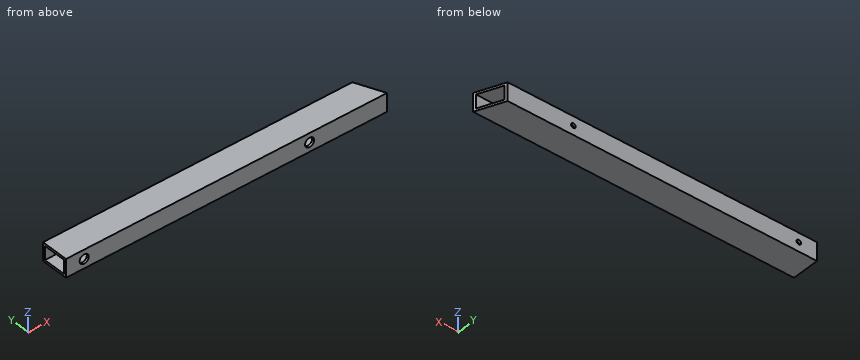
```python
from build123d import *

# Parameters (mm, degrees)
SKETCH1_W                 = 25.4
SKETCH1_H                 = 38.1
SKETCH1_W_2               = 19.05
SKETCH1_H_2               = 31.75
BEAM_DEPTH                = 447.675
MITER_CUT_DEPTH           = 449.799474292
SKETCH4_R                 = 3.175
BOLT_CLEARANCE_HOLE_DEPTH = 450.472808549
SKETCH5_R                 = 6.35
CLEARANCE_HOLE_DEPTH      = 12.7


with BuildPart() as part:
    # Sketch1 → beam (new body)
    with BuildSketch(Plane(origin=(0, 0, 0), x_dir=(0, 0, -1), z_dir=(1, 0, 0))):
        Rectangle(SKETCH1_W, SKETCH1_H)
        Rectangle(SKETCH1_W_2, SKETCH1_H_2, mode=Mode.SUBTRACT)
    extrude(amount=-BEAM_DEPTH)

    # Sketch2 → miter cut (cut, through all)
    with BuildSketch(Plane.XY.offset(12.7)):
        Polygon((0, -19.05), (-16.172490498, 19.05), (0, 19.05), align=None)
    extrude(amount=-MITER_CUT_DEPTH, mode=Mode.SUBTRACT)

    # Sketch4 → bolt clearance hole (cut, through all)
    with BuildSketch(Plane(origin=(0, 19.05, 0), x_dir=(1, 0, 0), z_dir=(0, 1, 0))):
        with Locations(Location((-422.275, 0, 0), (0, 0, 270))):
            Circle(SKETCH4_R)
        with Locations(Location((-107.95, 0, 0), (0, 0, 270))):
            Circle(SKETCH4_R)
    extrude(amount=-BOLT_CLEARANCE_HOLE_DEPTH, mode=Mode.SUBTRACT)

    # Sketch5 → clearance hole (cut)
    with BuildSketch(Plane.XZ.offset(19.05)):
        with Locations(Location((-422.275, 0, 0), (0, 0, 270))):
            Circle(SKETCH5_R)
        with Locations(Location((-107.95, 0, 0), (0, 0, 270))):
            Circle(SKETCH5_R)
    extrude(amount=-CLEARANCE_HOLE_DEPTH, mode=Mode.SUBTRACT)


solid = part.part
```
Part model, mm, in its own coordinate system. Give positions to 0.01 mm unless a question says otherwise; leave off trailing zeros. Order: outer loops, then holes, each group sorted by start corner. A loop starts at its lowest first (then second) coordinate and runs counter-clockwise, first axis right, second up. Notation, with made-up numbers: M 85.25,33.25 L 137.25,33.25 A8 cw 137.25,47.25 Z; hole C 6.25,-32 d8. An arc over 180 degrees is marked long. Use a Markdown table: item, result. Add a question column.
(1) Saw through at B-B, the plane y = 4. Give the cut face in (x, z) (3 decimals), and give its area (3 significant figures).
(2) Saw through at A-A, the plane x = -210. Give the cut face in (y, z) (3 decimals), and give its area (3 significant figures).
(3) Drop a flat-ended pin along its axis: P1, Ø5.5, axis at x = -422.275, z = 0, coming from the +Y side. Give the stop position or say it passes through.
(4) Probe line 1 along X through (y, z) = (18.25, 0) (3 decimals); line 2 along X through (y, z) = (18.4, 0) (3 decimals); line 3 along Z through (x, y) = (-132.5, 11.5) (3 decimals). List the from-to ranges inside material, lowest first. Write a range as [from, to].
Answer key:
| question | item | result |
|---|---|---|
| 1 | outline | M -447.675,-12.7 L -9.784,-12.7 L -9.784,-9.525 L -447.675,-9.525 Z; M -447.675,9.525 L -9.784,9.525 L -9.784,12.7 L -447.675,12.7 Z |
| 1 | area | 2,780 mm^2 |
| 2 | outline | M -19.05,-12.7 L 19.05,-12.7 L 19.05,12.7 L -19.05,12.7 Z; hole M -15.875,-9.525 L 15.875,-9.525 L 15.875,9.525 L -15.875,9.525 Z |
| 2 | area | 363 mm^2 |
| 3 | P1 | through |
| 4 | line 1 | [-447.675, -425.45], [-419.1, -111.125], [-104.775, -15.833] |
| 4 | line 2 | [-447.675, -425.45], [-419.1, -111.125], [-104.775, -15.897] |
| 4 | line 3 | [-12.7, -9.525], [9.525, 12.7] |
